Part model, mm, in its own coordinate system. A direction names the side the tool comes from. Round coordinates to 2 decimals unless told otherwise and drop trailing zeros. Loops run counter-clockwise (first coordinate to the right, second up) from the corner with the lowest first, then second, coordinate; pieces in that order, holes last. Notation, with made-up numbers: M 11,44 L 28,44 A22 cw 28,58 Z; hole C 19,45 d4. An arc over 180 degrees is marked long. Write each question's results on one line, items separated by ' | '.
from build123d import *

# Parameters (mm, degrees)
BOSS_EXTRUDE1_DEPTH = 2
SKETCH2_R           = 11
BOSS_EXTRUDE3_DEPTH = 2


with BuildPart() as part:
    # Sketch1 → Boss-Extrude1 (new body)
    with BuildSketch(Plane(origin=(0, 0, 0), x_dir=(1, 0, 0), z_dir=(0, 1, 0))):
        with BuildLine():
            Line((-50.675392178, 10), (-50.675392178, 25))
            ThreePointArc((-50.675392178, 25), (-45.675392178, 30), (-40.675392178, 25))
            Line((-40.675392178, 25), (-40.675392178, 10))
            Line((-40.675392178, 10), (-10.675392178, 10))
            Line((-10.675392178, 10), (-10.675392178, 24.667030171))
            ThreePointArc((-10.675392178, 24.667030171), (-5.847512802, 30.002770955), (-0.675392178, 25))
            Line((-0.675392178, 25), (-0.675392178, 10))
            ThreePointArc((-0.675392178, 10), (-2.139858272, 6.464466094), (-5.675392178, 5))
            Line((-5.675392178, 5), (-45.675392178, 5))
            ThreePointArc((-45.675392178, 5), (-49.210926084, 6.464466094), (-50.675392178, 10))
        make_face()
        with BuildLine():
            Line((-43.125392178, 25), (-43.125392178, 15))
            ThreePointArc((-43.125392178, 15), (-45.675392178, 12.45), (-48.225392178, 15))
            Line((-48.225392178, 15), (-48.225392178, 25))
            ThreePointArc((-48.225392178, 25), (-45.675392178, 27.55), (-43.125392178, 25))
        make_face(mode=Mode.SUBTRACT)
        with BuildLine():
            Line((-8.225392178, 25), (-8.225392178, 15))
            ThreePointArc((-8.225392178, 15), (-5.675392178, 12.45), (-3.125392178, 15))
            Line((-3.125392178, 15), (-3.125392178, 25))
            ThreePointArc((-3.125392178, 25), (-5.675392178, 27.55), (-8.225392178, 25))
        make_face(mode=Mode.SUBTRACT)
    extrude(amount=BOSS_EXTRUDE1_DEPTH)

    # Sketch2 → Boss-Extrude3 (add)
    with BuildSketch(Plane(origin=(0, 0, -5), x_dir=(-1, 0, 0), z_dir=(0, 0, -1))):
        with BuildLine():
            Line((19.297037413, 10.004378208), (19.297037413, 2))
            Line((19.297037413, 2), (31.622351713, 2))
            Line((31.622351713, 2), (31.622351713, 10.004378208))
            ThreePointArc((31.622351713, 10.004378208), (25.459694563, 33.379655531), (19.297037413, 10.004378208))
        make_face()
        with Locations((25.459694563, 20.879655531)):
            Circle(SKETCH2_R, mode=Mode.SUBTRACT)
    extrude(amount=BOSS_EXTRUDE3_DEPTH)


solid = part.part
Item 1: Band-saw the part on C-C on z = -26.75. Give the cut face in (x, y).
Filled sheet:
outline: M -50.36,0 L -47.53,0 L -47.53,2 L -50.36,2 Z; M -43.82,0 L -40.99,0 L -40.99,2 L -43.82,2 Z; M -10.37,0 L -7.53,0 L -7.53,2 L -10.37,2 Z; M -3.82,0 L -0.99,0 L -0.99,2 L -3.82,2 Z
Item 2: Drop flat-ended pins along their axis: P1, Ø1, axis at y = 7.5, z = -6, coming from the -X side; P2, Ø1, axis at x = -21.5, y = 0.5, coming from the -Z side; P3, Ø1.6, axis at y = 5.5, z = -6.5, coming from the +X side. Give the stop position or say it passes through.
Filled sheet:
P1: x = -31.62 | P2: z = -10 | P3: x = -19.3
Item 3: Band-saw the part on B-B on x = -47. Give the cut face in (y, z).
Filled sheet:
outline: M 0,-29.82 L 2,-29.82 L 2,-27.18 L 0,-27.18 Z; M 0,-12.82 L 2,-12.82 L 2,-5.18 L 0,-5.18 Z
Item 4: Wall check: L1, parallel to X at y = 14, z = -6.5; L2, parallel to Z at x = -32.5, y = 30; L3, parallel to Y at x = -31.5, z = -9.75. Give the ranges that are in metal, low to high.
Filled sheet:
L1: -35.9 to -34.04, -16.88 to -15.02 | L2: -7 to -5 | L3: 0 to 2
Item 5: Band-saw the part on D-D on x = -22. Give the cut face in (y, z).
Filled sheet:
outline: M 0,-10 L 2,-10 L 2,-7 L 10.44,-7 L 10.44,-5 L 0,-5 Z; M 31.32,-7 L 32.89,-7 L 32.89,-5 L 31.32,-5 Z
Item 6: Two-plate mould, pull along X, no slides. Class faces 1 (the flat face through (-0.675, 1, -18)), 2 (the cylindrical face through (-25.92, 33.37, -5.99)), 3 (the cylindrical face through (-5.62, 0.99, -27.55)): +X half, -X half, draft (parallel to the pull), parting line (faces both ways), or undercut.
Filled sheet:
face 1: +X half | face 2: parting line | face 3: undercut
Item 7: Band-saw the part on A-A on y = 14. Give the cut face in (x, z), and give its area (3 significant figures).
Filled sheet:
outline: M -35.9,-7 L -34.04,-7 L -34.04,-5 L -35.9,-5 Z; M -16.88,-7 L -15.02,-7 L -15.02,-5 L -16.88,-5 Z | area: 7.41 mm^2
Item 8: Which spindle directions (+Z, -Z, +X, -X, +Y, -Y) get a long thin tool onto all of the face, cutting with end or side? Do faces 4 (the cylindrical face through (-45.73, 0.99, -27.55)), 5 (the flat face through (-26, 1, -10)), 6 (the flat face through (-19.297, 6, -6)), 7 (the flat face through (-31.622, 6, -6)). Say none if no direction does.
Filled sheet:
face 4: +Y, -Y | face 5: -Z, +Y, -Y | face 6: +Z, -Z, +X | face 7: +Z, -Z, -X
